The model under review builds one solid part; all positions refer to its coordinate system, in mm. A direction names the side the tool comes from. Round coordinates to 2 decimals unless told otherwise and drop trailing zeros. Order: outer loops, then holes, each group sorted by start corner. A loop starts at its lowest first (then second) coordinate and runs counter-clockwise, first axis right, second up. Notation, with made-up numbers: M -38,12.5 L -17,12.5 A18 ccw -17,18.5 Z; hole C -16.5,76.5 d2. An arc over 180 degrees is marked long. One line per item, written item: value. Start each with the question number.
from build123d import *

# Parameters (mm, degrees)
BASE_FLANGE1_DEPTH          = 1.5
SM_EDGE_FLANGE_1_DEPTH      = 45
SM_EDGE_FLANGE_1_BEND_DEPTH = 45
SKETCH12_R                  = 3
CUT_EXTRUDE1_DEPTH          = 10
FILLET1_R                   = 10
SKETCH13_R                  = 3
CUT_EXTRUDE2_DEPTH          = 10
SKETCH14_R                  = 3
CUT_EXTRUDE3_DEPTH          = 10


# Sheet-metal steps are written as plain solids
with BuildPart() as part:
    # Sketch1 → Base-Flange1 (new body)
    with BuildSketch(Plane.XY):
        with BuildLine():
            Line((15, 0), (115, 0))
            ThreePointArc((115, 0), (125.606601718, 4.393398282), (130, 15))
            Line((130, 15), (130, 70))
            ThreePointArc((130, 70), (125.606601718, 80.606601718), (115, 85))
            Line((115, 85), (15, 85))
            ThreePointArc((15, 85), (4.393398282, 80.606601718), (0, 70))
            Line((0, 70), (0, 15))
            ThreePointArc((0, 15), (4.393398282, 4.393398282), (15, 0))
        make_face()
        with BuildLine():
            Line((104.5, 12.5), (25.5, 12.5))
            ThreePointArc((25.5, 12.5), (16.307611845, 16.307611845), (12.5, 25.5))
            Line((12.5, 25.5), (12.5, 59.5))
            ThreePointArc((12.5, 59.5), (16.307611845, 68.692388155), (25.5, 72.5))
            Line((25.5, 72.5), (104.5, 72.5))
            ThreePointArc((104.5, 72.5), (113.692388155, 68.692388155), (117.5, 59.5))
            Line((117.5, 59.5), (117.5, 25.5))
            ThreePointArc((117.5, 25.5), (113.692388155, 16.307611845), (104.5, 12.5))
        make_face(mode=Mode.SUBTRACT)
    extrude(amount=-BASE_FLANGE1_DEPTH)

    # Ребро-кромка1 section (across the edge) → Ребро-кромка1 (add)
    with BuildSketch(Plane(origin=(-0.76629509, 20, -1.5), x_dir=(0.7071067811865438, 0, -0.7071067811865512), z_dir=(0, 1, 0))):
        with BuildLine():
            Line((-1.5, 0.76629509), (-1.5, 49.378679656))
            Line((-1.5, 49.378679656), (0, 49.378679656))
            Line((0, 49.378679656), (0, 0.76629509))
            ThreePointArc((0, 0.76629509), (0.140822865, 0.058330741), (0.541852455, -0.541852455))
            Line((0.541852455, -0.541852455), (-0.518807717, -1.602512627))
            ThreePointArc((-0.518807717, -1.602512627), (-1.244996434, -0.515694408), (-1.5, 0.76629509))
        make_face()
    extrude(amount=SM_EDGE_FLANGE_1_DEPTH)

    # Ребро-кромка1 section 2 (across the edge) → Ребро-кромка1 bend (add)
    with BuildSketch(Plane(origin=(130.76629509, 65, -1.5), x_dir=(-0.7071067811865438, 0, -0.7071067811865512), z_dir=(0, -1, 0))):
        with BuildLine():
            Line((-1.5, 0.76629509), (-1.5, 49.378679656))
            Line((-1.5, 49.378679656), (0, 49.378679656))
            Line((0, 49.378679656), (0, 0.76629509))
            ThreePointArc((0, 0.76629509), (0.140822865, 0.058330741), (0.541852455, -0.541852455))
            Line((0.541852455, -0.541852455), (-0.518807717, -1.602512627))
            ThreePointArc((-0.518807717, -1.602512627), (-1.244996434, -0.515694408), (-1.5, 0.76629509))
        make_face()
    extrude(amount=SM_EDGE_FLANGE_1_BEND_DEPTH)

    # Sketch12 → Cut-Extrude1 (cut)
    with BuildSketch(Plane(origin=(65.693807717, 0, 65.693807717), x_dir=(0.7071067811865511, 0, -0.707106781186544), z_dir=(0.707106781186544, 0, 0.7071067811865511))):
        with Locations((134.905073837, 30)):
            Circle(SKETCH12_R)
        with Locations((134.905073837, 55)):
            Circle(SKETCH12_R)
    extrude(amount=-CUT_EXTRUDE1_DEPTH, mode=Mode.SUBTRACT)

    # Fillet1
    fillet1_edges = [part.edges().sort_by_distance(p)[0] for p in [
        (-36.212624407, 20, -35.885669145),
        (-36.212624407, 65, -35.885669145),
        (166.212624407, 65, -35.885669145),
        (166.212624407, 20, -35.885669145),
    ]]
    fillet(fillet1_edges, radius=FILLET1_R)

    # Sketch13 → Cut-Extrude2 (cut)
    with BuildSketch(Plane(origin=(-0.693807717, 0, 0.693807717), x_dir=(0.7071067811865511, 0, 0.707106781186544), z_dir=(-0.707106781186544, 0, 0.7071067811865511))):
        with Locations((-42.981192283, 30)):
            Circle(SKETCH13_R)
        with Locations((-42.981192283, 55)):
            Circle(SKETCH13_R)
    extrude(amount=-CUT_EXTRUDE2_DEPTH, mode=Mode.SUBTRACT)

    # Sketch14 → Cut-Extrude3 (cut)
    with BuildSketch(Plane(origin=(0, 0, -1.5), x_dir=(-1, 0, 0), z_dir=(0, 0, -1))):
        with Locations((-65, 6.25)):
            Circle(SKETCH14_R)
        with Locations((-65, 78.75)):
            Circle(SKETCH14_R)
    extrude(amount=-CUT_EXTRUDE3_DEPTH, mode=Mode.SUBTRACT)


solid = part.part
Item 1: Consider section A-A, the plane y = 47. Give the boundary of the cut face in (x, z).
Item 2: Consider section C-C, the plane x = 65. Give the boundary of the cut face in (y, z).
Item 3: Wall thickness on L1, parallel to Y at x = 65, z = -0.75; L2, parallel to Z at x = 119.5, y = 27.5; L3, parallel to X at y = 47, z = -30: over which ranges is each line inside the solid? List them lowest first.
Item 4: Clearance check with flat-ended pins moving along their axes: P1, Ø4, axis at y = 45.5, z = -20.5, coming from the +X side; P2, Ø1.7, axis at y = 18, z = -0.5, coming from the -X side; P3, Ø9, axis at x = -15, z = -15.5, coming from the +Y side; P4, Ø10, axis at x = 103.5, y = 9, coming from the +Z side. State where each tip first meets the part, or that it passes through.
Item 5: Machinability: for faces 1 (the cylindrical face through (125.72, 80.49, -0.74)), 2 (the cylindrical face through (113.793, 16.409, -0.74)), 3 (the flat face through (50, 5, -1.5)), which of the approach directions +Z, -Z, +X, -X, +Y, -Y give a long, thin tool a straight path to every point of the face, cutting with its end or side? Answer none if there is none.
Item 6: Consider section D-D, the plane z = -7. Give the boundary of the cut face in (x, y).
Item 7: Consider section B-B, the plane x = 28. Give the boundary of the cut face in (y, z).
Item 8: The part is to be moulded in two halves that separate along X. For faces 4 (the cylindrical face through (164.079, 22.852, -33.767)), 5 (the flat face through (-15, 20, -15)), 6 (the flat face through (-19.32, 42.18, -17.93)), 7 (the cylindrical face through (-30.839, 57.974, -30.498)), say which applies: pulls with the +X half, pulls with the -X half, needs draft (parallel to the pull), parting line crosses it, or undercut.
Computed:
1. outline: M -36.74,-35.36 L -35.68,-36.42 L -1.31,-2.04 A1.85 cw 0,-1.5 L 12.5,-1.5 L 12.5,0 L 0,0 A3.35 ccw -2.37,-0.98 Z; M 117.5,-1.5 L 130,-1.5 A1.85 cw 131.31,-2.04 L 165.68,-36.42 L 166.74,-35.36 L 132.37,-0.98 A3.35 ccw 130,0 L 117.5,0 Z
2. outline: M 0,-1.5 L 3.25,-1.5 L 3.25,0 L 0,0 Z; M 9.25,-1.5 L 12.5,-1.5 L 12.5,0 L 9.25,0 Z; M 72.5,-1.5 L 75.75,-1.5 L 75.75,0 L 72.5,0 Z; M 81.75,-1.5 L 85,-1.5 L 85,0 L 81.75,0 Z
3. L1: y = 0 to 3.25, 9.25 to 12.5, 72.5 to 75.75, 81.75 to 85
3. L2: z = -1.5 to 0
3. L3: x = -31.39 to -29.27, 159.27 to 161.39
4. P1: stops at x = 153.89
4. P2: stops at x = 0
4. P3: stops at y = 65
4. P4: stops at z = 0
5. face 1: +Z, -Z, +X, +Y
5. face 2: +Z, -Z
5. face 3: -Z, +Y, -Y
6. outline: M -8.39,20 L -6.27,20 L -6.27,65 L -8.39,65 Z; M 136.27,20 L 138.39,20 L 138.39,65 L 136.27,65 Z
7. outline: M 0,-1.5 L 12.5,-1.5 L 12.5,0 L 0,0 Z; M 72.5,-1.5 L 85,-1.5 L 85,0 L 72.5,0 Z
8. face 4: pulls with the +X half
8. face 5: needs draft
8. face 6: pulls with the -X half
8. face 7: undercut
